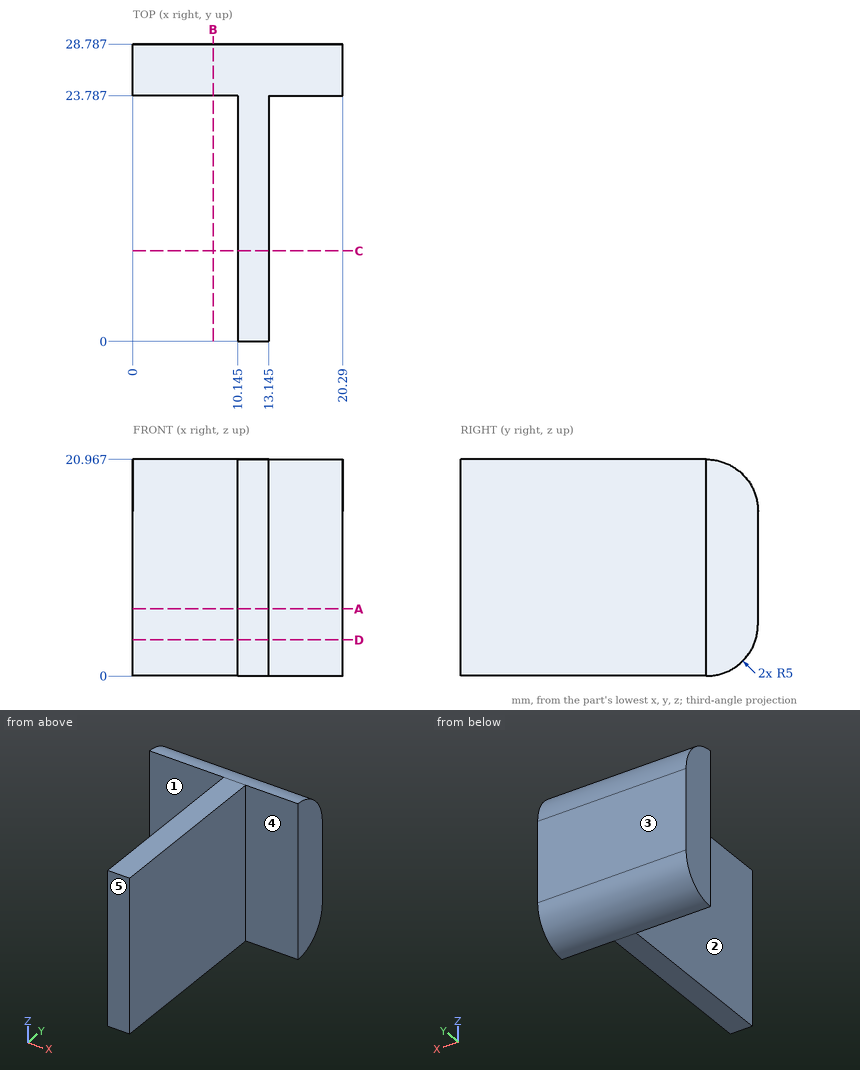
Check sheet for the drawn part. Datum: minimum x, y, z corner. Units: mm. A direction names the side the tool comes from. Give positions to 0.01 mm unless a question says otherwise; leave off trailing zeros. Write each loop counter-clockwise with the first axis right and the second up, starting at its lowest first coordinate (ties: lowest second). Pieces come first, ordered by that corner, then holes.
(1) Cross-section at D-D (z = 3.5). Enter the section's corners in (x, y) (1 decimal), plus the area to 3 significant figures.
(2) Material ranges on line 1 (Y direction, x = 18, z = 14.75); line 2 (X direction, y = 15, z = 18.75) (1 decimal); line 3 (Y direction, x = 6.75, z = 20.25) (1 decimal), recorded low to high.
(3) Cross-section at B-B (x = 7.75). Enter the section's corners in (y, z), plus the area to 3 significant figures.
(4) Mould release check, pull along Y, two halves, no side actions. Record for the marked faces 1, 2 and 3: +Y half, -Y half, draft (parallel to the pull), parting line (faces both ways), or undercut.
(5) Cross-section at C-C (y = 8.75). Enter the section's corners in (x, z) (1 decimal), plus the area to 3 significant figures.
(6) Access from +Z, -Z, +X, -X, +Y, -Y to the whole of each face (thin tool, end or side, straight path). Record for the marked faces 4 and 5.
(7) Gauge pin test, flat ends, axial feed: pin 1 (3 mm diameter, centred on y = 13, z = 13, fed in from -X) (3 decimals); pin 2 (5 mm diameter, centred on x = 5, z = 9, fed in from -Y); pin 3 (6.5 mm diameter, centred on y = 11.5, z = 14.5, fed in from +X) (3 decimals). Record the tip position at first contact, or that the pin passes through.
(8) Cross-section at A-A (z = 6.5). Enter the section's corners in (x, y) (1 decimal), plus the area to 3 significant figures.
Worked out:
1. outline: (0, 23.8) - (10.1, 23.8) - (10.1, 0) - (13.1, 0) - (13.1, 23.8) - (20.3, 23.8) - (20.3, 28.6) - (0, 28.6) - close
1. area: 168 mm2
2. line 1: y = 23.79 to 28.79
2. line 2: x = 10.1 to 13.1
2. line 3: y = 23.8 to 26.4
3. outline: (23.79, 0) arc R5 ccw to (28.79, 5) - (28.79, 15.97) arc R5 ccw to (23.79, 20.97) - close
3. area: 94.1 mm2
4. face 1: -Y half
4. face 2: draft
4. face 3: +Y half
5. outline: (10.1, 0) - (13.1, 0) - (13.1, 21) - (10.1, 21) - close
5. area: 62.9 mm2
6. face 4: +Z, -Z, +X, -Y
6. face 5: +Z, -Z, +X, -X, -Y
7. pin 1: stops at x = 10.145
7. pin 2: stops at y = 23.79
7. pin 3: stops at x = 13.145
8. outline: (0, 23.8) - (10.1, 23.8) - (10.1, 0) - (13.1, 0) - (13.1, 23.8) - (20.3, 23.8) - (20.3, 28.8) - (0, 28.8) - close
8. area: 173 mm2
